Design review of the part built by this model. Coordinates are the model's own, in mm. A direction names the side the tool comes from. Give positions to 0.01 mm unless a question says otherwise; leave off trailing zeros. Loops run counter-clockwise (first coordinate to the right, second up) from the corner with the lowest first, then second, coordinate; pieces in that order, holes last. Notation, with made-up numbers: M 18,-37 L 42,-37 A20 cw 42,-4 Z; hole C 67,-13 d1. An arc over 180 degrees is marked long. Use a Markdown table: item, result. Add a question column.
(1) For faces 4 (the face through (-4.336, 17.627, 19.524)), 5 (the face through (0.66, 1.042, -14.985)), 6 (the face through (1.846, 4.437, -39.599)), list the 3-axis set-ups (+Z, -Z, +X, -X, +Y, -Y) from which the entire face can be reached by the end or side of a thin tool; tool diameter is ignored.
(2) Add section A-A, the plane y = 51.5. Give the boundary of the cut face in (x, z), then the cut area to 3 significant figures.
(3) Add section B-B, the plane y = 42.5. Give the boundary of the cut face in (x, z).
(4) For probe 1 along Z at (x, y) = (0, 25); probe 2 along Y at (x, z) = (9.5, 29); probe 3 along Y at (x, z) = (-5, 16.5), list the stretches that pass through material, from the lowest coordinate up.
(5) Draft analysis for pull direction Z (two halves, no side actions). For faces 1 (the face through (0, 27, 13)), 2 (the face through (39.865, 4.437, 1.201)), 3 (the face through (26.327, -0.986, -10.916)), state which applies: pulls with the +Z half, pulls with the -Z half, needs draft (parallel to the pull), parting line crosses it, or undercut.
(6) Insertion check: pin 1 Ø6.5 at (x, z) = (-36.05, 0) entering from -Y; pin 2 Ø24 at (x, z) = (0, 0) entering from -Y; pin 3 Ø6 at (x, z) = (0, 0) entering from -Y; pin 4 Ø4 at (y, z) = (37, -0.5) entering from -X. Each pin has a flat end and moves straight along its axis. Give the tip position at first contact, or say it passes through.
```python
from build123d import *

# Parameters (mm, degrees)
SKETCH1_R           = 45
BOSS_EXTRUDE1_DEPTH = 9
SKETCH3_R           = 20
BOSS_EXTRUDE2_DEPTH = 18
SKETCH4_R           = 12.5
BOSS_EXTRUDE3_DEPTH = 28
SKETCH5_R           = 28.5
BOSS_EXTRUDE4_DEPTH = 2
SKETCH6_R           = 5
CUT_EXTRUDE1_DEPTH  = 40
CUT_EXTRUDE2_REACH  = 57
SKETCH8_R           = 4
CUT_EXTRUDE3_REACH  = 78.14
SKETCH9_R           = 2.5
CHAMFER1_SIZE       = 0.5


with BuildPart() as part:
    # Sketch1 → Boss-Extrude1 (new body)
    with BuildSketch(Plane(origin=(0, 0, 0), x_dir=(1, 0, 0), z_dir=(0, 1, 0))):
        Circle(SKETCH1_R)
    extrude(amount=BOSS_EXTRUDE1_DEPTH)

    # Sketch3 → Boss-Extrude2 (add)
    with BuildSketch(Plane(origin=(0, 9, 0), x_dir=(1, 0, 0), z_dir=(0, 1, 0))):
        Circle(SKETCH3_R)
    extrude(amount=BOSS_EXTRUDE2_DEPTH)

    # Sketch4 → Boss-Extrude3 (add)
    with BuildSketch(Plane(origin=(0, 27, 0), x_dir=(1, 0, 0), z_dir=(0, 1, 0))):
        Circle(SKETCH4_R)
    extrude(amount=BOSS_EXTRUDE3_DEPTH)

    # Sketch5 → Boss-Extrude4 (add)
    with BuildSketch(Plane.XZ):
        Circle(SKETCH5_R)
    extrude(amount=BOSS_EXTRUDE4_DEPTH)

    # Sketch6 → Cut-Extrude1 (cut)
    with BuildSketch(Plane(origin=(0, 55, 0), x_dir=(1, 0, 0), z_dir=(0, 1, 0))):
        Circle(SKETCH6_R)
    extrude(amount=-CUT_EXTRUDE1_DEPTH, mode=Mode.SUBTRACT)

    # Sketch7 → Cut-Revolve1 (revolve, cut)
    with BuildSketch(Plane(origin=(0, 0, 0), x_dir=(0, 0, -1), z_dir=(1, 0, 0))):
        with BuildLine():
            add(Edge.make_bspline(
                [(-15, 4), (-8.560208032, 11.204773426), (0, 13)],
                knots=[0, 0, 0, 1, 1, 1], degree=2))
            Line((0, 13), (0, -2))
            Line((0, -2), (-15, -2))
            Line((-15, -2), (-15, 4))
        make_face()
    revolve(axis=Axis((0, -2, 0), (0, 1, 0)), mode=Mode.SUBTRACT)

    # Sketch8 → Cut-Extrude2 (cut, up to next)
    with BuildSketch(Plane.XZ, mode=Mode.PRIVATE) as cut_extrude2_sk1:
        with Locations((0, 36.05)):
            Circle(SKETCH8_R)
    cut_extrude2_tool1 = extrude(cut_extrude2_sk1.sketch, amount=-CUT_EXTRUDE2_REACH, mode=Mode.PRIVATE) & part.part
    add(cut_extrude2_tool1.solids().sort_by_distance((0, 0, 36.05))[0], mode=Mode.SUBTRACT)
    # Sketch8 → Cut-Extrude2 (cut, up to next)
    with BuildSketch(Plane.XZ, mode=Mode.PRIVATE) as cut_extrude2_sk2:
        with Locations((-36.05, 0)):
            Circle(SKETCH8_R)
    cut_extrude2_tool2 = extrude(cut_extrude2_sk2.sketch, amount=-CUT_EXTRUDE2_REACH, mode=Mode.PRIVATE) & part.part
    add(cut_extrude2_tool2.solids().sort_by_distance((-36.05, 0, 0))[0], mode=Mode.SUBTRACT)
    # Sketch8 → Cut-Extrude2 (cut, up to next)
    with BuildSketch(Plane.XZ, mode=Mode.PRIVATE) as cut_extrude2_sk3:
        with Locations((0, -36.05)):
            Circle(SKETCH8_R)
    cut_extrude2_tool3 = extrude(cut_extrude2_sk3.sketch, amount=-CUT_EXTRUDE2_REACH, mode=Mode.PRIVATE) & part.part
    add(cut_extrude2_tool3.solids().sort_by_distance((0, 0, -36.05))[0], mode=Mode.SUBTRACT)
    # Sketch8 → Cut-Extrude2 (cut, up to next)
    with BuildSketch(Plane.XZ, mode=Mode.PRIVATE) as cut_extrude2_sk4:
        with Locations((36.05, 0)):
            Circle(SKETCH8_R)
    cut_extrude2_tool4 = extrude(cut_extrude2_sk4.sketch, amount=-CUT_EXTRUDE2_REACH, mode=Mode.PRIVATE) & part.part
    add(cut_extrude2_tool4.solids().sort_by_distance((36.05, 0, 0))[0], mode=Mode.SUBTRACT)

    # Sketch9 → Cut-Extrude3 (cut, up to next)
    with BuildSketch(Plane(origin=(8.838834765, 0, -8.838834765), x_dir=(0, -1, 0), z_dir=(-0.707106781, 0, 0.707106781)), mode=Mode.PRIVATE) as cut_extrude3_sk1:
        with Locations((-42.5, 0)):
            Circle(SKETCH9_R)
    cut_extrude3_tool1 = extrude(cut_extrude3_sk1.sketch, amount=CUT_EXTRUDE3_REACH, mode=Mode.PRIVATE) & part.part
    add(cut_extrude3_tool1.solids().sort_by_distance((8.838835, 42.5, -8.838835))[0], mode=Mode.SUBTRACT)

    # Chamfer1
    chamfer1_edges = [part.edges().sort_by_distance(p)[0] for p in [
        (-12.5, 55, 0),
        (-45, 9, 0),
        (-20, 27, 0),
    ]]
    chamfer(chamfer1_edges, length=CHAMFER1_SIZE)


solid = part.part
```
Established:
| question | item | result |
|---|---|---|
| 1 | face 4 | +Y |
| 1 | face 5 | -Y |
| 1 | face 6 | +Y, -Y |
| 2 | outline | C 0,0 d25; hole C 0,0 d10 |
| 2 | area | 412 mm^2 |
| 3 | outline | M 1.29,-4.83 A5 cw long 4.83,-1.29 L 10.43,-6.89 A12.5 ccw long 6.89,-10.43 Z |
| 4 | probe 1 | -20 to -5, 5 to 20 |
| 4 | probe 2 | 0 to 9 |
| 4 | probe 3 | -2 to 27 |
| 5 | face 1 | needs draft |
| 5 | face 2 | undercut |
| 5 | face 3 | parting line crosses it |
| 6 | pin 1 | through |
| 6 | pin 2 | y = 6.96 |
| 6 | pin 3 | y = 12.18 |
| 6 | pin 4 | x = -12.5 |
